The model under review builds one solid part; all positions refer to its coordinate system, in mm. Face numbers are marked on the shaded views. A direction names the side the tool comes from. Round coordinates to 2 decimals unless told otherwise and drop trailing zeros. Write each loop counter-clockwise with the first axis right and the second up, starting at its lowest first coordinate (ties: lowest second). Pieces come first, ordered by that corner, then holes. Notation, with made-up numbers: (16, 69.25) -> (55, 69.25) arc R19 ccw to (55, 79.25) -> close; hole circle Ø8 at (15.5, 64). An arc over 180 degrees is marked (long way). Return JSON: item names as keys, results as strings. Group by question number.
1. Tool access review of the marked faces 5 and 6: name each direction out of +Z, -Z, +X, -X, +Y, -Y from which nothing blocks a thin tool from reaching the whole face with its end or side.
2. Take a section at A-A, the plane y = 98.5. Write out the cut boundary in (x, z).
3. Take a section at B-B, the plane x = 129.5. Write out the cut boundary in (y, z).
4. For line 1 along Z through (x, y) = (330.5, -1.1) (3 decimals); line 2 along X through (y, z) = (-1.45, -305.88) (3 decimals); line 3 along Z through (x, y) = (351, 125), list the stretches that pass through material, from the lowest coordinate up. Write a range as from..to.
5. Clearance check with a flat-ended pin moving along its axis: P1, Ø2, axis at x = 188, z = -138.5, coming from the -Y side. State where the tip first meets the part, or that it passes through.
6. Mouldability with a two-part tool opening along Y and no side actions: class the marked faces 1, 2, 3 and 4 as pulls with the +Y half, pulls with the -Y half, needs draft (parallel to the pull), parting line crosses it, or undercut.
7. Take a section at C-C, the plane z = -154. Write out the cut boundary in (x, y), then the cut area to 3 significant figures.
from build123d import *

# Parameters (mm, degrees)
CROQUIS1_W              = 428
CROQUIS1_H              = 317
SALIENTE_EXTRUIR1_DEPTH = 1.9
CROQUIS3_W              = 428
CROQUIS3_H              = 1.9
SALIENTE_EXTRUIR2_DEPTH = 320.8
CROQUIS4_W              = 428
CROQUIS4_H              = 1.9
SALIENTE_EXTRUIR3_DEPTH = 317
CROQUIS6_W              = 428
CROQUIS6_H              = 1.9
SALIENTE_EXTRUIR4_DEPTH = 19.52
CROQUIS7_W              = 428
CROQUIS7_H              = 1.9
SALIENTE_EXTRUIR5_DEPTH = 73.52
CROQUIS8_R              = 3.175
CORTAR_EXTRUIR1_DEPTH   = 1.9


with BuildPart() as part:
    # Croquis1 → Saliente-Extruir1 (new body)
    with BuildSketch(Plane.XY):
        with Locations((214, 158.5)):
            Rectangle(CROQUIS1_W, CROQUIS1_H)
    extrude(amount=SALIENTE_EXTRUIR1_DEPTH)

    # Croquis3 → Saliente-Extruir2 (add)
    with BuildSketch(Plane.XY.offset(1.9)):
        with Locations((214, 317.95)):
            Rectangle(CROQUIS3_W, CROQUIS3_H)
    extrude(amount=-SALIENTE_EXTRUIR2_DEPTH)

    # Croquis4 → Saliente-Extruir3 (add)
    with BuildSketch(Plane.XZ.offset(-317)):
        with Locations((214, -317.95)):
            Rectangle(CROQUIS4_W, CROQUIS4_H)
    extrude(amount=SALIENTE_EXTRUIR3_DEPTH)

    # Croquis6 → Saliente-Extruir4 (add)
    with BuildSketch(Plane(origin=(0, 0, -318.9), x_dir=(-1, 0, 0), z_dir=(0, 0, -1))):
        with Locations((-214, -0.95)):
            Rectangle(CROQUIS6_W, CROQUIS6_H)
    extrude(amount=-SALIENTE_EXTRUIR4_DEPTH)

    # Croquis7 → Saliente-Extruir5 (add)
    with BuildSketch(Plane.XY.offset(1.9)):
        with Locations((214, -0.95)):
            Rectangle(CROQUIS7_W, CROQUIS7_H)
    extrude(amount=-SALIENTE_EXTRUIR5_DEPTH)

    # Croquis8 → Cortar-Extruir1 (cut)
    with BuildSketch(Plane.XZ.offset(1.9)):
        with Locations(Location((214, -305.88, 0), (0, 0, 270))):
            Circle(CROQUIS8_R)
        with Locations(Location((330.5, -305.88, 0), (0, 0, 270))):
            Circle(CROQUIS8_R)
        with Locations(Location((97.5, -305.88, 0), (0, 0, 270))):
            Circle(CROQUIS8_R)
        with Locations(Location((97.5, -65.12, 0), (0, 0, 270))):
            Circle(CROQUIS8_R)
        with Locations(Location((330.5, -65.12, 0), (0, 0, 270))):
            Circle(CROQUIS8_R)
        with Locations(Location((214, -65.12, 0), (0, 0, 270))):
            Circle(CROQUIS8_R)
    extrude(amount=-CORTAR_EXTRUIR1_DEPTH, mode=Mode.SUBTRACT)


solid = part.part
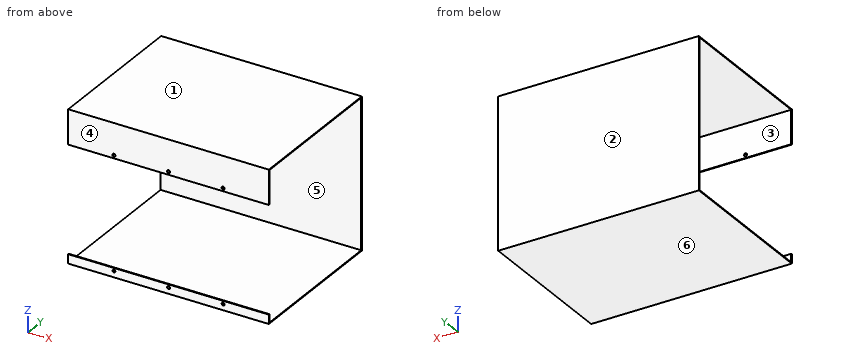
Output:
{
 "1": {"face 5": "+X, -X", "face 6": "-Z, +X, -X, +Y, -Y"},
 "2": {"outline": "(0, -318.9) -> (428, -318.9) -> (428, -317) -> (0, -317) -> close; (0, 0) -> (428, 0) -> (428, 1.9) -> (0, 1.9) -> close"},
 "3": {"outline": "(-1.9, -318.9) -> (318.9, -318.9) -> (318.9, 1.9) -> (-1.9, 1.9) -> (-1.9, -71.62) -> (0, -71.62) -> (0, 0) -> (317, 0) -> (317, -317) -> (0, -317) -> (0, -299.38) -> (-1.9, -299.38) -> close"},
 "4": {"line 1": "z = -318.9..-309.055, -302.705..-299.38, -71.62..-68.295, -61.945..1.9", "line 2": "x = 0..94.325, 100.675..210.825, 217.175..327.325, 333.675..428", "line 3": "z = -318.9..-317, 0..1.9"},
 "5": {"P1": "stops at y = 317"},
 "6": {"face 1": "needs draft", "face 2": "pulls with the +Y half", "face 3": "undercut", "face 4": "pulls with the -Y half"},
 "7": {"outline": "(0, 317) -> (428, 317) -> (428, 318.9) -> (0, 318.9) -> close", "area": "813 mm^2"}
}
